Source: CAD feature listing. Evaluate the final solid. Frame: model axes, mm. Face numbers are marked on the shaded views. A direction names the side the tool comes from. Give positions to 0.01 mm unless a question says otherwise; leave off trailing zeros. Write each loop counter-clockwise with the first axis right and the second up, starting at its lowest first coordinate (ties: lowest second). Pieces come first, ordered by that corner, then holes. Notation, with made-up numbers: (10.5, -28) -> (67.5, -28) arc R9 ccw to (67.5, -23) -> close; hole circle Ø3 at (6, -31.5). An arc over 180 degrees is marked (long way). Answer as a JSON object with one key per item and string values. Group by question number.
Item 1: Ray query, probe 1 along Y at (x, z) = (3.64, 1.3); probe 2 along Z at (x, y) = (1.5, 4.5); probe 3 along X at (y, z) = (-9.5, 8). Return the intervals inside material, ascending. Write a range as from..to.
Item 2: Section query D-D on y = -4. Return the cut outline in (x, z), plus the area to 3 significant figures.
Item 3: Section query A-A on z = 1. Return the cut outline in (x, y).
Item 4: Section query C-C on y = 3. Return the cut outline in (x, z).
Item 5: Pull-direction query (X, two-part tool) for the marked faces 4, 5, 6 and 7; classes: pulls with the +X half, pulls with the -X half, needs draft (parallel to the pull), parting line crosses it, or undercut.
Item 6: First-contact query: pin 1 Ø1.2 at (x, z) = (-12, 2.5) entering from +Y; pin 2 Ø3 at (y, z) = (4, 9.5) entering from +X; pin 3 Ø8 at (x, y) = (-12.5, 1.5) entering from +Z; pin 4 Ø2.5 at (x, y) = (7.28, 12) entering from +Z. Flat tips, straight axial feed; report the tip coordinate or a pass-through.
Item 7: Section query B-B on x = 7.28. Return the cut outline in (y, z).
Item 8: Access query for the marked faces 1, 2 and 3. Directions: +Z, -Z, +X, -X, +Y, -Y. A direction counts if a zero-diameter tool reaches every point of the face in a straight line with its end or side. Return the directions, or none.
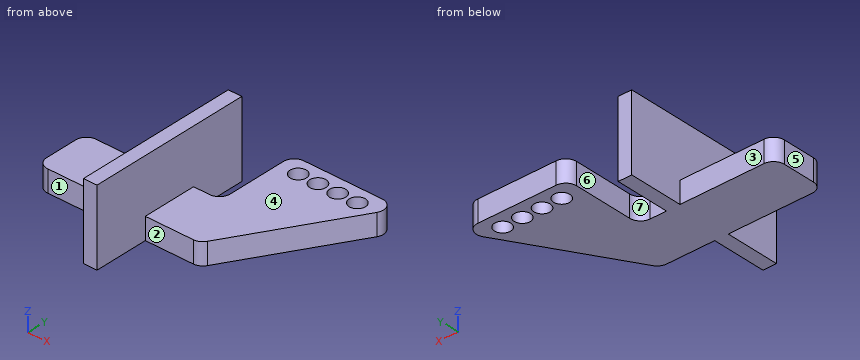
from build123d import *

# Parameters (mm, degrees)
ESQUISSE1_R        = 1.5
BOSS_EXTRU_1_DEPTH = 4
ESQUISSE2_W        = 2.5
ESQUISSE2_H        = 30
BOSS_EXTRU_2_DEPTH = 10
CONG_1_R           = 2


with BuildPart() as part:
    # Esquisse1 → Boss.-Extru.1 (new body)
    with BuildSketch(Plane.XY):
        Polygon((0, 0), (0, 15), (20, 15), (5, -10), (-5, -10), (-5, -20), (-7.5, -20), (-7.5, -10), (-25, -10), (-25, 0), (-7.5, 0), (-7.5, 10), (-5, 10), (-5, 0), align=None)
        with Locations((3.64, 12)):
            Circle(ESQUISSE1_R, mode=Mode.SUBTRACT)
        with Locations((7.28, 12)):
            Circle(ESQUISSE1_R, mode=Mode.SUBTRACT)
        with Locations((10.92, 12)):
            Circle(ESQUISSE1_R, mode=Mode.SUBTRACT)
        with Locations((14.56, 12)):
            Circle(ESQUISSE1_R, mode=Mode.SUBTRACT)
    extrude(amount=BOSS_EXTRU_1_DEPTH)

    # Esquisse2 → Boss.-Extru.2 (add)
    with BuildSketch(Plane.XY.offset(4)):
        with Locations((-6.25, -5)):
            Rectangle(ESQUISSE2_W, ESQUISSE2_H)
    extrude(amount=BOSS_EXTRU_2_DEPTH)

    # Congé1
    cong_1_edges = [part.edges().sort_by_distance(p)[0] for p in [
        (0, 0, 2),
        (0, 15, 2),
        (20, 15, 2),
        (5, -10, 2),
        (-25, -10, 2),
        (-25, 0, 2),
    ]]
    fillet(cong_1_edges, radius=CONG_1_R)


solid = part.part
Worked answers:
{
 "1": {"probe 1": "-10..10.5, 13.5..15", "probe 2": "0..4", "probe 3": "-7.5..-5"},
 "2": {"outline": "(-25, 0) -> (8.6, 0) -> (8.6, 4) -> (-5, 4) -> (-5, 14) -> (-7.5, 14) -> (-7.5, 4) -> (-25, 4) -> close", "area": "159 mm^2"},
 "3": {"outline": "(-25, -8) arc R2 ccw to (-23, -10) -> (-7.5, -10) -> (-7.5, -20) -> (-5, -20) -> (-5, -10) -> (3.87, -10) arc R2 ccw to (5.58, -9.03) -> (18.18, 11.97) arc R2 ccw to (16.47, 15) -> (2, 15) arc R2 ccw to (0, 13) -> (0, 2) arc R2 cw to (-2, 0) -> (-5, 0) -> (-5, 10) -> (-7.5, 10) -> (-7.5, 0) -> (-23, 0) arc R2 ccw to (-25, -2) -> close; hole circle Ø3 at (3.64, 12); hole circle Ø3 at (7.28, 12); hole circle Ø3 at (10.92, 12); hole circle Ø3 at (14.56, 12)"},
 "4": {"outline": "(-7.5, 0) -> (-5, 0) -> (-5, 14) -> (-7.5, 14) -> close; (0, 0) -> (12.8, 0) -> (12.8, 4) -> (0, 4) -> close"},
 "5": {"face 4": "needs draft", "face 5": "pulls with the -X half", "face 6": "undercut", "face 7": "undercut"},
 "6": {"pin 1": "y = 0", "pin 2": "x = -5", "pin 3": "z = 4", "pin 4": "through"},
 "7": {"outline": "(-6.2, 0) -> (10.5, 0) -> (10.5, 4) -> (-6.2, 4) -> close; (13.5, 0) -> (15, 0) -> (15, 4) -> (13.5, 4) -> close"},
 "8": {"face 1": "+Z, -Z, -X, -Y", "face 2": "+Z, -Z, +X, -Y", "face 3": "+Z, -Z, -X, +Y"}
}
